from build123d import *

# Parameters (mm, degrees)
SKETCH1_W           = 12
SKETCH1_H           = 25
SKETCH1_R           = 2.65
BOSS_EXTRUDE1_DEPTH = 6.5
FILLET1_R           = 1
CHAMFER1_SIZE       = 1


with BuildPart() as part:
    # Sketch1 → Boss-Extrude1 (new, symmetric)
    with BuildSketch(Plane(origin=(0, 0, 0), x_dir=(1, 0, 0), z_dir=(0, 1, 0))):
        Rectangle(SKETCH1_W, SKETCH1_H)
        with Locations(Location((0, 7.5, 0), (0, 0, 90))):
            Circle(SKETCH1_R, mode=Mode.SUBTRACT)
        with Locations(Location((0, -7.5, 0), (0, 0, 90))):
            Circle(SKETCH1_R, mode=Mode.SUBTRACT)
    extrude(amount=BOSS_EXTRUDE1_DEPTH, both=True)

    # Fillet1
    fillet1_edges = [part.edges().sort_by_distance(p)[0] for p in [
        (6, 0, 12.5),
        (-6, 0, 12.5),
        (-6, 0, -12.5),
        (6, 0, -12.5),
    ]]
    fillet(fillet1_edges, radius=FILLET1_R)

    # Chamfer1
    chamfer1_edges = [part.edges().sort_by_distance(p)[0] for p in [
        (0, 6.5, 12.5),
        (-6, 6.5, 0),
        (6, 6.5, 0),
        (0, 6.5, -12.5),
        (5.707106781, 6.5, 12.207106781),
        (5.707106781, 6.5, -12.207106781),
        (-5.707106781, 6.5, -12.207106781),
        (-5.707106781, 6.5, 12.207106781),
    ]]
    chamfer(chamfer1_edges, length=CHAMFER1_SIZE)


solid = part.part
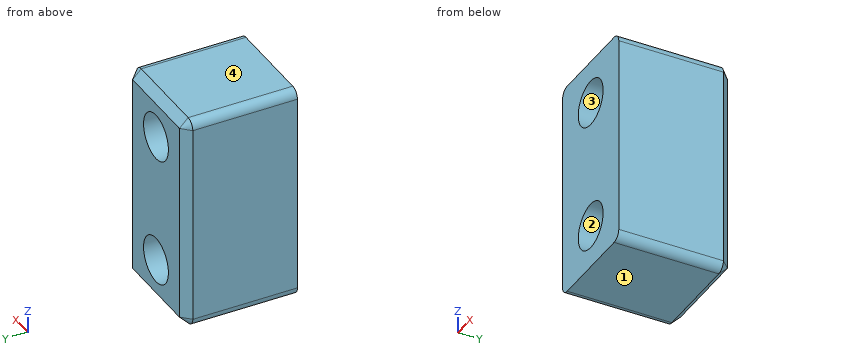
Read the model definition and answer for the solid it produces. Units are mm, in the model's axes. Face numbers are marked on the shaded views. Round coordinates to 2 decimals unless told otherwise and drop trailing zeros. Write each loop counter-clockwise with the first axis right and the second up, starting at its lowest first coordinate (ties: lowest second). Pieces come first, ordered by that corner, then holes. Notation, with made-up numbers: M 36,14.5 L 73,14.5 A8 cw 73,21.5 Z; hole C 32.5,0.5 d10. An arc over 180 degrees is marked long. Use a Markdown table: item, result.
1) The part is cut by section C-C (y = 1.25). Write down the section's boundary in (x, z).
Answers follow:
| item | result |
|---|---|
| outline | M -6,-11.5 A1 ccw -5,-12.5 L 5,-12.5 A1 ccw 6,-11.5 L 6,11.5 A1 ccw 5,12.5 L -5,12.5 A1 ccw -6,11.5 Z; hole C 0,-7.5 d5.3; hole C 0,7.5 d5.3 |
2) The part is cut by section B-B (z = -7.5). Write down the section's boundary in (x, y).
Answers follow:
| item | result |
|---|---|
| outline | M -6,-6.5 L -2.65,-6.5 L -2.65,6.5 L -5,6.5 L -6,5.5 Z; M 2.65,-6.5 L 6,-6.5 L 6,5.5 L 5,6.5 L 2.65,6.5 Z |
3) The part is cut by section A-A (x = 0). Write down the section's boundary in (y, z), plus the area to 3 significant figures.
Answers follow:
| item | result |
|---|---|
| outline | M -6.5,-12.5 L 5.5,-12.5 L 6.5,-11.5 L 6.5,-10.15 L -6.5,-10.15 Z; M -6.5,-4.85 L 6.5,-4.85 L 6.5,4.85 L -6.5,4.85 Z; M -6.5,10.15 L 6.5,10.15 L 6.5,11.5 L 5.5,12.5 L -6.5,12.5 Z |
| area | 186 mm2 |
4) The part is cut by section D-D (x = -2.25). Write down the section's boundary in (y, z), plus the area to 3 significant figures.
Answers follow:
| item | result |
|---|---|
| outline | M -6.5,-12.5 L 5.5,-12.5 L 6.5,-11.5 L 6.5,-8.9 L -6.5,-8.9 Z; M -6.5,-6.1 L 6.5,-6.1 L 6.5,6.1 L -6.5,6.1 Z; M -6.5,8.9 L 6.5,8.9 L 6.5,11.5 L 5.5,12.5 L -6.5,12.5 Z |
| area | 251 mm2 |
5) For a pull along Z with two mould halves and no side action, classify the marked faces 1, 2, 3 and 4 as pulls with the +Z half, pulls with the -Z half, needs draft (parallel to the pull), parting line crosses it, or undercut.
Answers follow:
| item | result |
|---|---|
| face 1 | pulls with the -Z half |
| face 2 | undercut |
| face 3 | undercut |
| face 4 | pulls with the +Z half |
6) Straight lines are drawn through the part: line 1 along X through (y, z) = (-1.75, -7.5); line 2 along Z through (x, y) = (-0.25, 3.5); line 3 along Z through (x, y) = (-2, -3.5). For each, find the intervals that lie inside material, in ascending order. Write a range as [from, to].
Answers follow:
| item | result |
|---|---|
| line 1 | x = [-6, -2.65], [2.65, 6] |
| line 2 | z = [-12.5, -10.14], [-4.86, 4.86], [10.14, 12.5] |
| line 3 | z = [-12.5, -9.24], [-5.76, 5.76], [9.24, 12.5] |
